Read the model definition and answer for the solid it produces. Units are mm, in the model's axes. Face numbers are marked on the shaded views. A direction names the side the tool comes from. Round coordinates to 2 decimals unless told otherwise and drop trailing zeros. Order: outer loops, then holes, each group sorted by start corner. A loop starts at its lowest first (then second) coordinate and runs counter-clockwise, first axis right, second up. Notation, with made-up numbers: (42.5, 81.5) - (86.5, 81.5) arc R17 cw to (86.5, 89.5) - close; hole circle Ø1 at (-20, -35). An arc over 180 degrees is marked (long way). Answer as a JSON object with one key per item and string values. Group by question number.
Q1. Consider line 1 (Z direction, x = -19.75, y = 1.75); line 2 (Z direction, x = -17.5, y = 5.5); line 3 (Z direction, x = -10.75, y = -0.25). Determine where each line is inside the solid, lowest interval first.
Q2. A cutting plane is placed at B-B on z = -12. Determine the outline of the cut face in (x, y), and give its area (3 significant figures).
Q3. A tool of negligible diameter and unlimited length cuts with its end or side. For the marked faces 1 and 2, from which of +Z, -Z, +X, -X, +Y, -Y can it reach the whole face along a straight path? Write none if from no direction.
Q4. A cutting plane is placed at C-C on x = -12.5. Count the separate pieces of the cut face and the enclosed holes in it, and give its area (3 significant figures).
Q5. The mould has two halves that part along Z. Classify the marked faces 3, 4, 5 and 6: pulls with the +Z half, pulls with the -Z half, needs draft (parallel to the pull), parting line crosses it, or undercut.
Q6. Given pin 1 Ø2.5 at (x, y) = (-7, 0) entering from +Z; pin 2 Ø0.8 at (x, z) = (-6.5, 0.5) entering from -Y; pin 3 Ø1.7 at (x, z) = (-23, 1) entering from -Y; pin 4 Ø11 at (x, z) = (-15.81, -2.69) entering from -Y (3 decimals), each flat-ended and moving along its own axis, determine where each tip first touches the part or whether it passes through.
Q7. A cutting plane is placed at A-A on x = -6.5. Determine the outline of the cut face in (y, z).
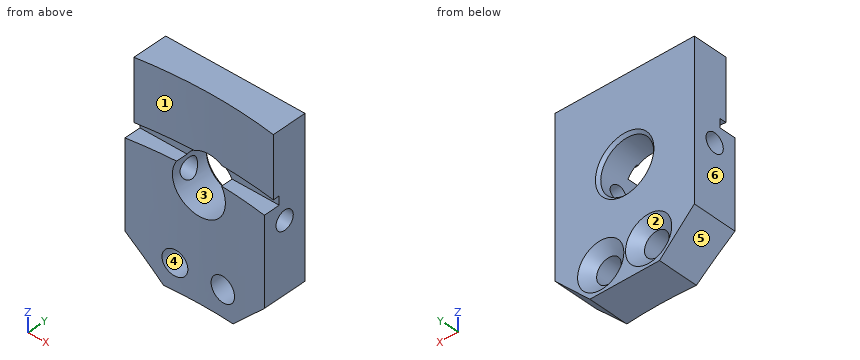
```python
from build123d import *

# Parameters (mm, degrees)
BOSS_EXTRUDE1_DEPTH                               = 6.35
CUT_EXTRUDE1_DEPTH                                = 46.530235335
CUT_EXTRUDE1_DEPTH_BACK                           = 46.530235335
SKETCH2_R                                         = 83.82
BOSS_EXTRUDE2_DEPTH                               = 22.225
CHAMFER1_SIZE                                     = 6.35
CSK_FOR_8_FLAT_HEAD_MACHINE_SCREW_100_D           = 4.4958
CSK_FOR_8_FLAT_HEAD_MACHINE_SCREW_100_CSINK_D     = 8.4328
CSK_FOR_8_FLAT_HEAD_MACHINE_SCREW_100_CSINK_ANGLE = 100
SKETCH6_R                                         = 1.524
CUT_EXTRUDE2_DEPTH                                = 38.145162749
SKETCH7_W                                         = 1.5875
SKETCH7_H                                         = 2.989850087
CUT_EXTRUDE3_DEPTH                                = 35.437066375
SKETCH8_R                                         = 4.826
CUT_EXTRUDE4_DEPTH                                = 38.145162749
CHAMFER2_SIZE                                     = 0.508
F_8_32_TAPPED_HOLE1_D                             = 3.4544


with BuildPart() as part:
    # Sketch1 → Boss-Extrude1 (new body)
    with BuildSketch(Plane(origin=(0, 0, 0), x_dir=(1, 0, 0), z_dir=(0, 1, 0))):
        Polygon((-28.511825699, 16.020271113), (-22.161825699, 22.370271113), (-9.461825699, 22.370271113), (-3.111825699, 16.020271113), (-3.111825699, -12.554728887), (-28.511825699, -12.554728887), align=None)
    extrude(amount=BOSS_EXTRUDE1_DEPTH)

    # Sketch2 → Cut-Extrude1 (cut, two sides: drawn at the far end of the back side and taken through both)
    with BuildSketch(Plane.XY.offset(12.554728887).offset(-CUT_EXTRUDE1_DEPTH_BACK)):
        with Locations((-15.811825699, -82.852292666)):
            Circle(SKETCH2_R)
    extrude(amount=CUT_EXTRUDE1_DEPTH + CUT_EXTRUDE1_DEPTH_BACK, mode=Mode.SUBTRACT)

    # Sketch5 → Boss-Extrude2 (add)
    with BuildSketch(Plane(origin=(0, 0, -22.370271113), x_dir=(-1, 0, 0), z_dir=(0, 0, -1))):
        with BuildLine():
            Line((3.111825699, 6.35), (3.111825699, 0))
            Line((3.111825699, 0), (3.111825699, -1.799225087))
            ThreePointArc((3.111825699, -1.799225087), (15.811825699, -0.810292666), (28.511825699, -1.799225087))
            Line((28.511825699, -1.799225087), (28.511825699, 0))
            Line((28.511825699, 0), (28.511825699, 6.35))
            Line((28.511825699, 6.35), (3.111825699, 6.35))
        make_face()
    extrude(amount=-BOSS_EXTRUDE2_DEPTH)

    # Chamfer1
    chamfer1_edges = [part.edges().sort_by_distance(p)[0] for p in [
        (-3.111825699, 2.275387457, -22.370271113),
        (-28.511825699, 2.275387457, -22.370271113),
    ]]
    chamfer(chamfer1_edges, length=CHAMFER1_SIZE)

    # CSK for #8 Flat Head Machine Screw (100)1 (through all)
    with Locations(Plane(origin=(0, 6.35, 0), x_dir=(1, 0, 0), z_dir=(0, 1, 0))):
        with Locations((-20.177450699, 17.607771113), (-11.446200699, 17.607771113)):
            CounterSinkHole(CSK_FOR_8_FLAT_HEAD_MACHINE_SCREW_100_D / 2, CSK_FOR_8_FLAT_HEAD_MACHINE_SCREW_100_CSINK_D / 2, counter_sink_angle=CSK_FOR_8_FLAT_HEAD_MACHINE_SCREW_100_CSINK_ANGLE)

    # Sketch6 → Cut-Extrude2 (cut, through all)
    with BuildSketch(Plane(origin=(0, 6.35, 0), x_dir=(1, 0, 0), z_dir=(0, 1, 0))):
        with Locations(Location((-15.811825699, 2.685271113, 0), (0, 0, 270))):
            Circle(SKETCH6_R)
    extrude(amount=-CUT_EXTRUDE2_DEPTH, mode=Mode.SUBTRACT)

    # Sketch7 → Cut-Extrude3 (cut, through all)
    with BuildSketch(Plane(origin=(-3.111825699, 0, 0), x_dir=(0, 0, -1), z_dir=(1, 0, 0))):
        with Locations((-0.648478887, -0.304300044)):
            Rectangle(SKETCH7_W, SKETCH7_H)
    extrude(amount=-CUT_EXTRUDE3_DEPTH, mode=Mode.SUBTRACT)

    # Sketch8 → Cut-Extrude4 (cut, through all)
    with BuildSketch(Plane(origin=(0, 6.35, 0), x_dir=(1, 0, 0), z_dir=(0, 1, 0))):
        with Locations(Location((-15.811825699, 2.685271113, 0), (0, 0, 270))):
            Circle(SKETCH8_R)
    extrude(amount=-CUT_EXTRUDE4_DEPTH, mode=Mode.SUBTRACT)

    # Chamfer2
    chamfer2_edges = [part.edges().sort_by_distance(p)[0] for p in [
        (-15.811825699, 6.35, -7.511271113),
    ]]
    chamfer(chamfer2_edges, length=CHAMFER2_SIZE)

    # #8-32 Tapped Hole1 (through all)
    with Locations(Plane.ZY.offset(28.511825699)):
        with Locations((-3.320271113, 2.275387457)):
            Hole(F_8_32_TAPPED_HOLE1_D / 2)


solid = part.part
```
Result set:
{
 "1": {"line 1": "z = -22.37 to -19.81, -15.4 to -5.47, 0.1 to 12.55", "line 2": "z = -22.37 to -19.37, -15.85 to -7.21, 1.84 to 12.55", "line 3": "z = -22.37 to -19.75, -15.47 to -0.15"},
 "2": {"outline": "(-28.51, -1.8) arc R82.04 cw to (-3.11, -1.8) - (-3.11, 6.35) - (-28.51, 6.35) - close", "area": "190 mm²"},
 "3": {"face 1": "+Z, -Y", "face 2": "+Y"},
 "4": {"separate pieces": "3", "enclosed holes": "0", "area": "148 mm²"},
 "5": {"face 3": "undercut", "face 4": "undercut", "face 5": "pulls with the -Z half", "face 6": "needs draft"},
 "6": {"pin 1": "stops at z = 12.55", "pin 2": "stops at y = 1.19", "pin 3": "stops at y = 0.59", "pin 4": "stops at y = -0.995"},
 "7": {"outline": "(-1.34, -19.41) - (6.35, -19.41) - (6.35, 12.55) - (0.45, 12.55) - (0.45, 1.44) - (1.19, 1.44) - (1.19, -0.15) - (-1.34, -0.15) - close; hole circle Ø3.45 at (2.28, -3.32)"}
}
